```python
from build123d import *

# Parameters (mm, degrees)
SKETCH1_W           = 64
SKETCH1_H           = 110
BOSS_EXTRUDE1_DEPTH = 1.5
SKETCH2_W           = 6
SKETCH2_H           = 4.5
BOSS_EXTRUDE2_DEPTH = 13.1
BOSS_EXTRUDE3_DEPTH = 2.65
BOSS_EXTRUDE4_DEPTH = 3.35
SKETCH7_R           = 1
CUT_EXTRUDE1_DEPTH  = 6


with BuildPart() as part:
    # Sketch1 → Boss-Extrude1 (new body)
    with BuildSketch(Plane(origin=(0, 0, 0), x_dir=(1, 0, 0), z_dir=(0, 1, 0))):
        Rectangle(SKETCH1_W, SKETCH1_H)
    extrude(amount=BOSS_EXTRUDE1_DEPTH)

    # Sketch2 → Boss-Extrude2 (add)
    with BuildSketch(Plane(origin=(0, 1.5, 0), x_dir=(1, 0, 0), z_dir=(0, 1, 0))):
        with Locations((-25.75, 40.15)):
            Rectangle(SKETCH2_W, SKETCH2_H)
    boss_extrude2 = extrude(amount=BOSS_EXTRUDE2_DEPTH)

    # Sketch3 → Boss-Extrude3 (add)
    with BuildSketch(Plane.ZY.offset(28.75)):
        Polygon((-42.4, 7.75), (-47.325, 4.625), (-52.25, 4.625), (-52.25, 1.5), (-42.4, 1.5), align=None)
        Polygon((-37.9, 14.6), (-24.8, 1.5), (-37.9, 1.5), align=None)
    boss_extrude3 = extrude(amount=-BOSS_EXTRUDE3_DEPTH)

    # Sketch6 → Boss-Extrude4 (add)
    with BuildSketch(Plane(origin=(-26.1, 0, 0), x_dir=(0, 0, -1), z_dir=(1, 0, 0))):
        Polygon((24.8, 1.5), (37.9, 1.5), (37.9, 14.6), align=None)
    boss_extrude4 = extrude(amount=BOSS_EXTRUDE4_DEPTH)

    # Sketch7 → Cut-Extrude1 (cut)
    with BuildSketch(Plane.ZY.offset(28.75)):
        with Locations((-40.15, 11.35)):
            Circle(SKETCH7_R)
    cut_extrude1 = extrude(amount=-CUT_EXTRUDE1_DEPTH, mode=Mode.SUBTRACT)

    # Mirror1: Boss-Extrude2, Boss-Extrude3, Boss-Extrude4, Cut-Extrude1 across plane
    add(boss_extrude2.mirror(Plane(origin=(0, 0, 0), x_dir=(0, 0, 1), z_dir=(1, 0, 0))))
    add(boss_extrude3.mirror(Plane(origin=(0, 0, 0), x_dir=(0, 0, 1), z_dir=(1, 0, 0))))
    add(boss_extrude4.mirror(Plane(origin=(0, 0, 0), x_dir=(0, 0, 1), z_dir=(1, 0, 0))))
    add(cut_extrude1.mirror(Plane(origin=(0, 0, 0), x_dir=(0, 0, 1), z_dir=(1, 0, 0))), mode=Mode.SUBTRACT)


solid = part.part
```
Build history of the part. All positions in model axes, mm. A direction names the side the tool comes from. Give positions to 0.01 mm unless a question says otherwise; leave off trailing zeros. Loops run counter-clockwise (first coordinate to the right, second up) from the corner with the lowest first, then second, coordinate; pieces in that order, holes last. Notation, with made-up numbers: (40.25, 35) -> (58.25, 35) arc R17 cw to (58.25, 68) -> close; hole circle Ø1 at (25, 53). An arc over 180 degrees is marked (long way). One line per question, with ' | ' between items.
Q1. Drop flat-ended pins along their axis: pin 1 (4 mm diameter, centred on y = 5.5, z = -37.5, fed in from +X); pin 2 (6.5 mm diameter, centred on y = 8.5, z = -29.5, fed in from -X); pin 3 (10 mm diameter, centred on x = 22, z = 5.5, fed in from +Y). Give the stop position or say it passes through.
Filled sheet:
pin 1: stops at x = 28.75 | pin 2: stops at x = -28.75 | pin 3: stops at y = 1.5
Q2. Pull direction Y, two halves, no side cores. Call faces 1 (the flat face through (-27, 3, -52.25)), 2 (the flat face through (25.8, 8.1, -31.4)), 3 (the cylindrical face through (-25.79, 11.39, -41.15)): pulls with the +Y half, pulls with the -Y half, needs draft (parallel to the pull), parting line crosses it, or undercut.
Filled sheet:
face 1: needs draft | face 2: pulls with the +Y half | face 3: undercut
Q3. Cut at B-B, the plane z = -29. Write the cut outline in (x, y), plus the area to 3 significant figures.
Filled sheet:
outline: (-32, 0) -> (32, 0) -> (32, 1.5) -> (28.75, 1.5) -> (28.75, 5.7) -> (22.75, 5.7) -> (22.75, 1.5) -> (-22.75, 1.5) -> (-22.75, 5.7) -> (-28.75, 5.7) -> (-28.75, 1.5) -> (-32, 1.5) -> close | area: 146 mm²
Q4. Cut at D-D, the plane z = 4. Write the cut outline in (x, y).
Filled sheet:
outline: (-32, 0) -> (32, 0) -> (32, 1.5) -> (-32, 1.5) -> close
Q5. Cut at A-A, the plane y = 3.5. Write the cut outline in (x, z).
Filled sheet:
outline: (-28.75, -52.25) -> (-26.1, -52.25) -> (-26.1, -42.4) -> (-22.75, -42.4) -> (-22.75, -26.8) -> (-28.75, -26.8) -> close; (22.75, -42.4) -> (26.1, -42.4) -> (26.1, -52.25) -> (28.75, -52.25) -> (28.75, -26.8) -> (22.75, -26.8) -> close
Q6. Cut at C-C, the plane x = 9. Write the cut outline in (y, z).
Filled sheet:
outline: (0, -55) -> (1.5, -55) -> (1.5, 55) -> (0, 55) -> close
Q7. Drill centre lines: line 1 along Y through (x, z) = (25.15, -40.15); line 2 along X through (y, z) = (5.5, -31.5); line 3 along Y through (x, z) = (-23, 37.5). Where is each one in solid material? Low to high. Write a range as [from, to].
Filled sheet:
line 1: y = [0, 10.35], [12.35, 14.6] | line 2: x = [-28.75, -22.75], [22.75, 28.75] | line 3: y = [0, 1.5]
Q8. Tool access for faces 4 (the flat face through (-28.75, 7, -39)), 5 (the flat face through (25, 9, -42.4)), 6 (the flat face through (27, 4.625, -50)), 7 (the flat face through (22.75, 7, -35)): list every direction of +Z, -Z, +X, -X, +Y, -Y with a clear straight run to the whole face (end or side of a thin tool).
Filled sheet:
face 4: +Z, -Z, -X, +Y | face 5: -Z, +Y | face 6: -Z, +X, -X, +Y | face 7: +Z, -Z, +Y
